Autodesk Fusion 360 part; units mm, degrees
sketch "Sketch2" plane through (0, 0, 0) normal (0, 1, 0) x (1, 0, 0)
  line L0 (0, 0) -> (31.75, 0)
  line L1 (31.75, 0) -> (31.75, -9.525)
  line L2 (31.75, -9.525) -> (0, -9.525)
  line L3 (0, -9.525) -> (0, 0)
  circle A0 centre (19.05, -4.7625) radius 2.1
  line L4 (23.8125, 0) -> (14.2875, 0)
  line L5 (14.2875, 0) -> (14.2875, -9.525)
  line L6 (14.2875, -9.525) -> (23.8125, -9.525)
  line L7 (23.8125, -9.525) -> (23.8125, 0)
  line L8 (23.8125, 0) -> (14.2875, -9.525) construction
  line L9 (14.2875, 0) -> (23.8125, -9.525) construction
  line L10 (0, -4) -> (14.2875, -4)
  line L11 (23.8125, -4) -> (31.75, -4)
  point P0 (19.05, -4.7625)
  dimension "d1" = 31.75
  dimension "d2" = 9.525
  dimension "d3" = 4.2
  dimension "d4" = 4.7625
  dimension "d5" = 19.05
  dimension "d8" = 9.525
  dimension "d9" = 9.525
  dimension "d10" = 4
  dimension "d11" = 4
extrude "Extrude1" add sketch "Sketch2" along normal blind 38.1 contours L0 L3 L5 L10 | L0 L2 L4 L5 L6 L7 | L0 L1 L7 L11
fillet "Fillet1" radius 4.7625 2 edges at (14.2875, 19.05, 9.525) (23.8125, 19.05, 9.525)
sketch "Sketch3" plane through (0, 0, 4) normal (0, 0, 1) x (-1, 0, 0)
  line L0 (0, 0) -> (-14.2875, 0)
  line L1 (-14.2875, 0) -> (-14.2875, -38.1)
  line L2 (-14.2875, -38.1) -> (0, -38.1)
  line L3 (0, -38.1) -> (0, 0)
sketch "Sketch4" plane through (0, 0, 4) normal (0, 0, 1) x (-1, 0, 0)
sketch "Sketch5" plane through (0, 0, 4) normal (0, 0, 1) x (-1, 0, 0)
  line L0 (-14.2875, -38.1) -> (0, -38.1) construction
  line L1 (0, -38.1) -> (0, 0) construction
  line L2 (0, 0) -> (-14.2875, 0) construction
  line L3 (-14.2875, 0) -> (-14.2875, -38.1) construction
  line L4 (-7.1437, -38.1) -> (-7.1437, 0) construction
  line L5 (-7.1437, -27.2901) -> (0, -27.2901) construction
  line L6 (-7.1437, -27.2901) -> (-14.2875, -27.2901) construction
  line L7 (-5.4299, -28.1) -> (-8.8576, -28.1)
  arc A0 (-8.8576, -28.1) -> (-8.8576, -33.1) centre (-8.8576, -30.6) ccw
  line L8 (-8.8576, -33.1) -> (-5.4299, -33.1)
  arc A1 (-5.4299, -33.1) -> (-5.4299, -28.1) centre (-5.4299, -30.6) ccw
  line L9 (-5.4299, -30.6) -> (-8.8576, -30.6) construction
  line L10 (-5.4437, -5) -> (-8.8438, -5)
  arc A2 (-8.8438, -5) -> (-8.8438, -10) centre (-8.8438, -7.5) ccw
  line L11 (-8.8438, -10) -> (-5.4437, -10)
  arc A3 (-5.4437, -10) -> (-5.4437, -5) centre (-5.4437, -7.5) ccw
  line L12 (-5.4437, -7.5) -> (-8.8438, -7.5) construction
  point P0 (0, -38.1)
  point P1 (-14.2875, -38.1)
  point P2 (-14.2875, 0)
  point P3 (-7.1437, -30.6)
  point P4 (-7.1438, -7.5)
  dimension "d14" = 5
  dimension "d16" = 5
  dimension "d19" = 7.5
  dimension "d20" = 7.5
extrude "Extrude2" cut sketch "Sketch5" against normal blind 4
Input: part model. Units: mm. Frame: model coordinates. A direction names the side the tool comes from. Coordinates: 2 decimals unless noted, no trailing zeros. Loops run counter-clockwise (first coordinate to the right, second up) from the corner with the lowest first, then second, coordinate; pieces in that order, holes last.
Q1. Cut plane C-C (x = 10). Output: boundary loops of the cut face in (y, z).
Q2. Cut plane B-B (z = 2.25). Output: boundary loops of the cut face in (x, y).
Q3. Cut plane A-A (y = 30.6). Give the number of separate pieces and of enclosed holes in the cut face, then the cut area to 3 significant figures.
Q4. Material intervals for line 1 (Z direction, x = 19, y = 29); line 2 (X direction, y = 27, z = 4.75); line 3 (Y direction, x = 11, z = 3), sorted ascending.
Q5. Draft query along Z for faces 1 (the face through (28, 19, 4)), 2 (the face through (7, 28.1, 2)), 3 (the face through (16.95, 18.78, 4.85)). Return one class per face: +Z half, -Z half, draft (parallel to the pull), parting line (faces both ways), or undercut.
Q6. Set-up query: faces 4 (the face through (7, 19, 4)), 5 (the face through (16, 19, 0)), 6 (the face through (11.357, 30.545, 2.028)). Return all of +Z, -Z, +X, -X, +Y, -Y with unobstructed straight access to the full face (end or side cutting, diameter ignored); none if empty.
Q7. Contact query for flat-ended pins moving along their axis: pin 1 (0.8 mm diameter, centred on y = 14.5, z = 4.5, fed in from +X); pin 2 (6 mm diameter, centred on x = 9, y = 23.5, fed in from +Z); pin 3 (5 mm diameter, centred on x = 16, y = 22.5, fed in from +Z). Output: stop coordinate, or through.
Working result:
1. outline: (0, 0) - (5.28, 0) - (5.28, 4) - (0, 4) - close; (9.72, 0) - (28.38, 0) - (28.38, 4) - (9.72, 4) - close; (32.82, 0) - (38.1, 0) - (38.1, 4) - (32.82, 4) - close
2. outline: (0, 0) - (31.75, 0) - (31.75, 38.1) - (0, 38.1) - close; hole (5.43, 28.1) - (8.86, 28.1) arc R2.5 ccw to (8.86, 33.1) - (5.43, 33.1) arc R2.5 ccw to start; hole (5.44, 5) - (8.84, 5) arc R2.5 ccw to (8.84, 10) - (5.44, 10) arc R2.5 ccw to start
3. separate pieces: 2
3. enclosed holes: 1
3. area: 122 mm2
4. line 1: z = 0 to 2.66, 6.86 to 9.52
4. line 2: x = 14.29 to 16.95, 21.15 to 23.81
4. line 3: y = 0 to 6.23, 8.77 to 29.31, 31.89 to 38.1
5. face 1: +Z half
5. face 2: draft
5. face 3: undercut
6. face 4: +Z, -X, +Y, -Y
6. face 5: -Z, +X, -X, +Y, -Y
6. face 6: +Z, -Z
7. pin 1: stops at x = 23.81
7. pin 2: stops at z = 4
7. pin 3: stops at z = 9.49
